from build123d import *

# Parameters (mm, degrees)
F2_DEPTH = 0.2
F3_DEPTH = 1


with BuildPart() as f2:
    # F0 (on Top) → F2 (new body)
    with BuildSketch(Plane.XY):
        with BuildLine():
            ThreePointArc((7, 3), (6.707107, 3.707107), (6, 4))
            Line((6, 4), (-6, 4))
            ThreePointArc((-6, 4), (-6.707107, 3.707107), (-7, 3))
            Line((-7, 3), (-7, -3))
            ThreePointArc((-7, -3), (-6.707107, -3.707107), (-6, -4))
            Line((-6, -4), (6, -4))
            ThreePointArc((6, -4), (6.707107, -3.707107), (7, -3))
            Line((7, -3), (7, 3))
        make_face()
    extrude(amount=F2_DEPTH)

    # F1 (on face) → F3 (cut)
    with BuildSketch(Plane.XY):
        with BuildLine():
            Line((5, 3), (-5, 3))
            ThreePointArc((-5, 3), (-5.707107, 2.707107), (-6, 2))
            Line((-6, 2), (-6, -2))
            ThreePointArc((-6, -2), (-5.707107, -2.707107), (-5, -3))
            Line((-5, -3), (5, -3))
            ThreePointArc((5, -3), (5.707107, -2.707107), (6, -2))
            Line((6, -2), (6, 2))
            ThreePointArc((6, 2), (5.707107, 2.707107), (5, 3))
        make_face()
    extrude(amount=F3_DEPTH, mode=Mode.SUBTRACT)


solid = f2.part
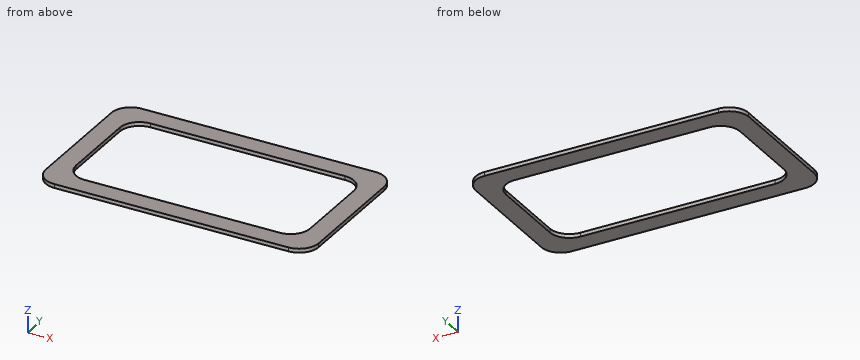
Part model, mm, in its own coordinate system. Coordinates: 2 decimals unless noted, no trailing zeros. Loops run counter-clockwise (first coordinate to the right, second up) from the corner with the lowest first, then second, coordinate; pieces in that order, holes last. Notation, with made-up numbers: (26, 0) - (47, 0) arc R15 ccw to (47, 28) - close; hole circle Ø2 at (-1.75, 51). An arc over 180 degrees is marked (long way). Write each question's results on one line, items separated by ' | '. Start each with the question number.
Q1. Slice it at C-C on y = -2.75. Give the cut face in (x, z), and give its area (3 significant figures).
Q2. Drop a flat-ended pin along its axis: pin 1 Ø3 at (x, y) = (2, 1) entering from -Z. Give the stop position or say it passes through.
Q3. Slice it at A-A on x = 1.5. Give the cut face in (y, z).
Q4. Slice it at B-B on z = 0.15. Give the cut face in (x, y), and give its area (3 significant figures).
Q5. Probe line 1 along Y through (x, z) = (3.25, 0.1); line 2 along X through (y, z) = (0, 0.1); line 3 along Y through (x, z) = (-5.75, 0.05). List the from-to ranges inside material, lowest first.
Answer:
1) outline: (-7, 0) - (-5.66, 0) - (-5.66, 0.2) - (-7, 0.2) - close; (5.66, 0) - (7, 0) - (7, 0.2) - (5.66, 0.2) - close | area: 0.535 mm2
2) pin 1: passes through
3) outline: (-4, 0) - (-3, 0) - (-3, 0.2) - (-4, 0.2) - close; (3, 0) - (4, 0) - (4, 0.2) - (3, 0.2) - close
4) outline: (-7, -3) arc R1 ccw to (-6, -4) - (6, -4) arc R1 ccw to (7, -3) - (7, 3) arc R1 ccw to (6, 4) - (-6, 4) arc R1 ccw to (-7, 3) - close; hole (-6, -2) arc R1 ccw to (-5, -3) - (5, -3) arc R1 ccw to (6, -2) - (6, 2) arc R1 ccw to (5, 3) - (-5, 3) arc R1 ccw to (-6, 2) - close | area: 40.0 mm2
5) line 1: y = -4 to -3, 3 to 4 | line 2: x = -7 to -6, 6 to 7 | line 3: y = -4 to -2.66, 2.66 to 4
